Design review of the part built by this model. Coordinates are the model's own, in mm. A direction names the side the tool comes from. Give positions to 0.01 mm unless a question says otherwise; leave off trailing zeros. Write each loop counter-clockwise with the first axis right and the second up, starting at its lowest first coordinate (ties: lowest second). Pieces come first, ordered by that corner, then holes. Notation, with made-up numbers: (68, 22) - (114, 22) arc R17 cw to (114, 28) - close; hole circle Ø3 at (-2, 78.25). An arc over 180 degrees is marked (long way). Write each question's results on one line, items separated by ' | '. Start each with the question number.
from build123d import *

# Parameters (mm, degrees)
EXTRUDE_1_DEPTH             = 5.5
SKETCH_2_R                  = 20
EXTRUDE_2_DEPTH             = 2
CHAMFER_1_SIZE              = 1.5
CHAMFER_1_SIZE2             = 1.787630389
CHAMFER_1_OF_MIRROR_1_SIZE2 = 1.5
CHAMFER_1_OF_MIRROR_1_SIZE  = 1.787630389
SKETCH_3_R                  = 3.4
CUT_EXTRUDE_1_DEPTH         = 30
SKETCH_8_R                  = 20
EXTRUDE_3_DEPTH             = 9
SKETCH_11_R                 = 33
EXTRUDE_4_DEPTH             = 90
SKETCH_10_R                 = 7.8
CUT_EXTRUDE_2_DEPTH         = 191
CHAMFER_2_SIZE              = 1
FILLET_1_R                  = 2


with BuildPart() as part:
    # 스케치1 → 보스-돌출1 (new, symmetric)
    with BuildSketch(Plane.XY):
        with BuildLine():
            Line((12.279067203, 9.260056493), (13.72951471, 11.331510209))
            ThreePointArc((13.72951471, 11.331510209), (13.819231237, 11.644886966), (13.696740348, 11.946963163))
            ThreePointArc((13.696740348, 11.946963163), (12.880233507, 12.823034344), (12.007805037, 13.643432236))
            ThreePointArc((12.007805037, 13.643432236), (11.644638313, 13.792108644), (11.267252957, 13.684521298))
            Line((11.267252957, 13.684521298), (9.202645163, 12.238867358))
            ThreePointArc((9.202645163, 12.238867358), (8.915071795, 12.148443996), (8.627783828, 12.239770064))
            ThreePointArc((8.627783828, 12.239770064), (7.516754209, 12.951796446), (6.347354905, 13.563248531))
            ThreePointArc((6.347354905, 13.563248531), (6.081851507, 13.807041329), (6.003955886, 14.158977765))
            Line((6.003955886, 14.158977765), (6.224353416, 16.678133059))
            ThreePointArc((6.224353416, 16.678133059), (6.145361829, 16.994383555), (5.888243509, 17.194743772))
            ThreePointArc((5.888243509, 17.194743772), (4.743092252, 17.54519025), (3.577348088, 17.81946143))
            ThreePointArc((3.577348088, 17.81946143), (3.188498275, 17.766635614), (2.915466643, 17.484769561))
            Line((2.915466643, 17.484769561), (1.850290815, 15.200492627))
            ThreePointArc((1.850290815, 15.200492627), (1.646456756, 14.978397074), (1.351995179, 14.913843704))
            ThreePointArc((1.351995179, 14.913843704), (0.033801995, 14.974961851), (-1.284653671, 14.919795238))
            ThreePointArc((-1.284653671, 14.919795238), (-1.636482757, 14.998174295), (-1.879910562, 15.26401238))
            Line((-1.879910562, 15.26401238), (-2.948618349, 17.555863625))
            ThreePointArc((-2.948618349, 17.555863625), (-3.175152318, 17.790248795), (-3.498003423, 17.835206672))
            ThreePointArc((-3.498003423, 17.835206672), (-4.664956742, 17.566126596), (-5.811656393, 17.220780324))
            ThreePointArc((-5.811656393, 17.220780324), (-6.121997301, 16.980606919), (-6.217516604, 16.599987941))
            Line((-6.217516604, 16.599987941), (-5.997847464, 14.089158172))
            ThreePointArc((-5.997847464, 14.089158172), (-6.06332522, 13.794900649), (-6.286059898, 13.591765005))
            ThreePointArc((-6.286059898, 13.591765005), (-7.458207642, 12.985598321), (-8.572440333, 12.27859486))
            ThreePointArc((-8.572440333, 12.27859486), (-8.916322788, 12.170558572), (-9.260056493, 12.279067203))
            Line((-9.260056493, 12.279067203), (-11.331510209, 13.72951471))
            ThreePointArc((-11.331510209, 13.72951471), (-11.644886966, 13.819231237), (-11.946963163, 13.696740348))
            ThreePointArc((-11.946963163, 13.696740348), (-12.823034344, 12.880233507), (-13.643432236, 12.007805037))
            ThreePointArc((-13.643432236, 12.007805037), (-13.792108644, 11.644638313), (-13.684521298, 11.267252957))
            Line((-13.684521298, 11.267252957), (-12.238867358, 9.202645163))
            ThreePointArc((-12.238867358, 9.202645163), (-12.148443996, 8.915071795), (-12.239770064, 8.627783828))
            ThreePointArc((-12.239770064, 8.627783828), (-12.951796446, 7.516754209), (-13.563248531, 6.347354905))
            ThreePointArc((-13.563248531, 6.347354905), (-13.807041329, 6.081851507), (-14.158977765, 6.003955886))
            Line((-14.158977765, 6.003955886), (-16.678133059, 6.224353416))
            ThreePointArc((-16.678133059, 6.224353416), (-16.994383555, 6.145361829), (-17.194743772, 5.888243509))
            ThreePointArc((-17.194743772, 5.888243509), (-17.54519025, 4.743092252), (-17.81946143, 3.577348088))
            ThreePointArc((-17.81946143, 3.577348088), (-17.766635614, 3.188498275), (-17.484769561, 2.915466643))
            Line((-17.484769561, 2.915466643), (-15.200492627, 1.850290815))
            ThreePointArc((-15.200492627, 1.850290815), (-14.978397015, 1.646456653), (-14.913843726, 1.351994942))
            ThreePointArc((-14.913843726, 1.351994942), (-14.974961851, 0.033801876), (-14.919795238, -1.284653671))
            ThreePointArc((-14.919795238, -1.284653671), (-14.998174295, -1.636482757), (-15.26401238, -1.879910562))
            Line((-15.26401238, -1.879910562), (-17.555863625, -2.948618349))
            ThreePointArc((-17.555863625, -2.948618349), (-17.790248795, -3.175152318), (-17.835206672, -3.498003423))
            ThreePointArc((-17.835206672, -3.498003423), (-17.566126596, -4.664956742), (-17.220780324, -5.811656393))
            ThreePointArc((-17.220780324, -5.811656393), (-16.980606919, -6.121997301), (-16.599987941, -6.217516604))
            Line((-16.599987941, -6.217516604), (-14.089158172, -5.997847464))
            ThreePointArc((-14.089158172, -5.997847464), (-13.794900649, -6.06332522), (-13.591765005, -6.286059898))
            ThreePointArc((-13.591765005, -6.286059898), (-12.985598321, -7.458207642), (-12.27859486, -8.572440333))
            ThreePointArc((-12.27859486, -8.572440333), (-12.170558572, -8.916322788), (-12.279067203, -9.260056493))
            Line((-12.279067203, -9.260056493), (-13.72951471, -11.331510209))
            ThreePointArc((-13.72951471, -11.331510209), (-13.819231237, -11.644886966), (-13.696740348, -11.946963163))
            ThreePointArc((-13.696740348, -11.946963163), (-12.880233507, -12.823034344), (-12.007805037, -13.643432236))
            ThreePointArc((-12.007805037, -13.643432236), (-11.644638313, -13.792108644), (-11.267252957, -13.684521298))
            Line((-11.267252957, -13.684521298), (-9.202645163, -12.238867358))
            ThreePointArc((-9.202645163, -12.238867358), (-8.915071795, -12.148443996), (-8.627783828, -12.239770064))
            ThreePointArc((-8.627783828, -12.239770064), (-7.516754209, -12.951796446), (-6.347354905, -13.563248531))
            ThreePointArc((-6.347354905, -13.563248531), (-6.081851507, -13.807041329), (-6.003955886, -14.158977765))
            Line((-6.003955886, -14.158977765), (-6.224353416, -16.678133059))
            ThreePointArc((-6.224353416, -16.678133059), (-6.145361829, -16.994383555), (-5.888243509, -17.194743772))
            ThreePointArc((-5.888243509, -17.194743772), (-4.743092252, -17.54519025), (-3.577348088, -17.81946143))
            ThreePointArc((-3.577348088, -17.81946143), (-3.188498275, -17.766635614), (-2.915466643, -17.484769561))
            Line((-2.915466643, -17.484769561), (-1.850290815, -15.200492627))
            ThreePointArc((-1.850290815, -15.200492627), (-1.646456653, -14.978397015), (-1.351994942, -14.913843726))
            ThreePointArc((-1.351994942, -14.913843726), (-0.033801876, -14.974961851), (1.284653671, -14.919795238))
            ThreePointArc((1.284653671, -14.919795238), (1.636482757, -14.998174295), (1.879910562, -15.26401238))
            Line((1.879910562, -15.26401238), (2.948618349, -17.555863625))
            ThreePointArc((2.948618349, -17.555863625), (3.175152318, -17.790248795), (3.498003423, -17.835206672))
            ThreePointArc((3.498003423, -17.835206672), (4.664956742, -17.566126596), (5.811656393, -17.220780324))
            ThreePointArc((5.811656393, -17.220780324), (6.121997301, -16.980606919), (6.217516604, -16.599987941))
            Line((6.217516604, -16.599987941), (5.997847464, -14.089158172))
            ThreePointArc((5.997847464, -14.089158172), (6.06332522, -13.794900649), (6.286059898, -13.591765005))
            ThreePointArc((6.286059898, -13.591765005), (7.458207642, -12.985598321), (8.572440333, -12.27859486))
            ThreePointArc((8.572440333, -12.27859486), (8.916322788, -12.170558572), (9.260056493, -12.279067203))
            Line((9.260056493, -12.279067203), (11.331510209, -13.72951471))
            ThreePointArc((11.331510209, -13.72951471), (11.644886966, -13.819231237), (11.946963163, -13.696740348))
            ThreePointArc((11.946963163, -13.696740348), (12.823034344, -12.880233507), (13.643432236, -12.007805037))
            ThreePointArc((13.643432236, -12.007805037), (13.792108644, -11.644638313), (13.684521298, -11.267252957))
            Line((13.684521298, -11.267252957), (12.238867358, -9.202645163))
            ThreePointArc((12.238867358, -9.202645163), (12.148443996, -8.915071914), (12.239769926, -8.627784023))
            ThreePointArc((12.239769926, -8.627784023), (12.951796386, -7.516754312), (13.563248531, -6.347354905))
            ThreePointArc((13.563248531, -6.347354905), (13.807041329, -6.081851507), (14.158977765, -6.003955886))
            Line((14.158977765, -6.003955886), (16.678133059, -6.224353416))
            ThreePointArc((16.678133059, -6.224353416), (16.994383555, -6.145361829), (17.194743772, -5.888243509))
            ThreePointArc((17.194743772, -5.888243509), (17.54519025, -4.743092252), (17.81946143, -3.577348088))
            ThreePointArc((17.81946143, -3.577348088), (17.766635614, -3.188498275), (17.484769561, -2.915466643))
            Line((17.484769561, -2.915466643), (15.200492627, -1.850290815))
            ThreePointArc((15.200492627, -1.850290815), (14.978397015, -1.646456653), (14.913843726, -1.351994942))
            ThreePointArc((14.913843726, -1.351994942), (14.974961851, -0.033801876), (14.919795238, 1.284653671))
            ThreePointArc((14.919795238, 1.284653671), (14.998174295, 1.636482757), (15.26401238, 1.879910562))
            Line((15.26401238, 1.879910562), (17.555863625, 2.948618349))
            ThreePointArc((17.555863625, 2.948618349), (17.790248795, 3.175152318), (17.835206672, 3.498003423))
            ThreePointArc((17.835206672, 3.498003423), (17.566126596, 4.664956742), (17.220780324, 5.811656393))
            ThreePointArc((17.220780324, 5.811656393), (16.980606919, 6.121997301), (16.599987941, 6.217516604))
            Line((16.599987941, 6.217516604), (14.089158172, 5.997847464))
            ThreePointArc((14.089158172, 5.997847464), (13.794900649, 6.06332522), (13.591765005, 6.286059898))
            ThreePointArc((13.591765005, 6.286059898), (12.985598253, 7.458207762), (12.278594702, 8.572440559))
            ThreePointArc((12.278594702, 8.572440559), (12.170558572, 8.916322926), (12.279067203, 9.260056493))
        make_face()
    extrude(amount=EXTRUDE_1_DEPTH, both=True)

    # 스케치2 → 보스-돌출2 (add)
    with BuildSketch(Plane.XY.offset(5.5)):
        Circle(SKETCH_2_R)
    extrude_2 = extrude(amount=EXTRUDE_2_DEPTH)

    # 모따기1
    chamfer_1_edges = [part.edges().sort_by_distance(p)[0] for p in [
        (-20, 0, 5.5),
    ]]
    chamfer_1_side = [part.faces().sort_by_distance(p)[0] for p in [
        (-20, 0, 6.5),
    ]]
    chamfer(chamfer_1_edges, length=CHAMFER_1_SIZE, length2=CHAMFER_1_SIZE2, reference=chamfer_1_side[0])

    # 대칭 복사1: 보스-돌출2 across plane
    add(extrude_2.mirror(Plane.XY))

    # 모따기1 of 대칭 복사1
    chamfer_1_of_mirror_1_edges = [part.edges().sort_by_distance(p)[0] for p in [
        (-20, 0, -5.5),
    ]]
    chamfer(chamfer_1_of_mirror_1_edges, length=CHAMFER_1_OF_MIRROR_1_SIZE, length2=CHAMFER_1_OF_MIRROR_1_SIZE2)

    # 스케치3 → 컷-돌출1 (cut)
    with BuildSketch(Plane(origin=(0, 0, -7.5), x_dir=(-1, 0, 0), z_dir=(0, 0, -1))):
        Circle(SKETCH_3_R)
    extrude(amount=-CUT_EXTRUDE_1_DEPTH, mode=Mode.SUBTRACT)

    # 스케치8 → 보스-돌출3 (add)
    with BuildSketch(Plane(origin=(0, 0, -7.5), x_dir=(-1, 0, 0), z_dir=(0, 0, -1))):
        with Locations(Location((0, 0, 0), (0, 0, 180))):
            Circle(SKETCH_8_R)
    extrude(amount=EXTRUDE_3_DEPTH)

    # 스케치11 → 보스-돌출4 (add)
    with BuildSketch(Plane(origin=(0, 0, -16.5), x_dir=(-1, 0, 0), z_dir=(0, 0, -1))):
        with Locations(Location((0, 0, 0), (0, 0, 180))):
            Circle(SKETCH_11_R)
    extrude(amount=EXTRUDE_4_DEPTH)

    # 스케치10 → 컷-돌출2 (cut)
    with BuildSketch(Plane.XY.offset(7.5)):
        Circle(SKETCH_10_R)
    extrude(amount=-CUT_EXTRUDE_2_DEPTH, mode=Mode.SUBTRACT)

    # 모따기2
    chamfer_2_edges = [part.edges().sort_by_distance(p)[0] for p in [
        (-7.8, 0, 7.5),
        (-7.8, 0, -106.5),
    ]]
    chamfer(chamfer_2_edges, length=CHAMFER_2_SIZE)

    # 필렛1
    fillet_1_edges = [part.edges().sort_by_distance(p)[0] for p in [
        (-33, 0, -16.5),
        (-33, 0, -106.5),
    ]]
    fillet(fillet_1_edges, radius=FILLET_1_R)


solid = part.part
Q1. Machinability: for faces 1 (the face through (0.052, 14.975, 0.077)), 2 (the face through (14.975, -0.052, 0.077)), 3 (the face through (-14.975, 0.052, 0.077)), which of the approach directions +Z, -Z, +X, -X, +Y, -Y give a long, thin tool a straight path to every point of the face, cutting with its end or side? Answer none if there is none.
Q2. The part is to be moulded in two halves that separate along X. For faces 4 (the face through (17.57, 4.65, 0.08)), 5 (the face through (-0.4, 20.2, -16.5)), 6 (the face through (-7.442, 12.995, 0.077)), say which applies: +X half, -X half, draft (parallel to the pull), parting line (faces both ways), or undercut.
Q3. Insertion check: P1, Ø2, axis at y = 15, z = -56, coming from the +X side; P2, Ø4, axis at y = -20, z = -58.5, coming from the +X side; P3, Ø2, axis at x = 21.5, y = 24, coming from the -Z side. Each pin has a flat end and moves straight along its axis. Give the tip position at first contact, or say it passes through.
Q4. For line 1 along Z through (x, y) = (15, 6.5); line 2 along Y through (x, z) = (0, -63); line 3 along X through (y, z) = (0.5, -90.5), list the stretches that pass through material, from the lowest coordinate up. Write a range as [from, to].
Q5. Add section C-C on z = -35.5. State the section outline as (x, y) points.
Result:
1) face 1: +Y | face 2: +X | face 3: -X
2) face 4: +X half | face 5: draft | face 6: undercut
3) P1: stops at x = 29.88 | P2: stops at x = 27.66 | P3: stops at z = -106.49
4) line 1: z = [-106.5, -5.5], [5.5, 7.5] | line 2: y = [-33, -7.8], [7.8, 33] | line 3: x = [-33, -7.78], [7.78, 33]
5) outline: circle Ø66 at (0, 0); hole circle Ø15.6 at (0, 0)
